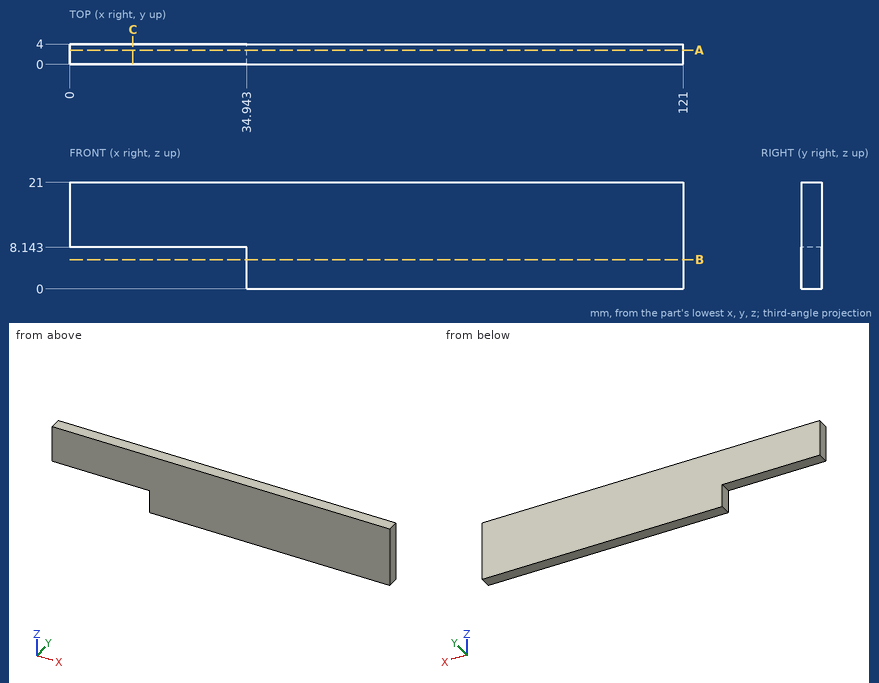
Here's the drawing with two shaded views (mm, measured from the low corner). I have some questions. Coordinates: 2 decimals unless noted, no trailing zeros. Write each loop counter-clockwise with the first axis right and the second up, starting at its lowest first coordinate (ties: lowest second). Pieces come first, ordered by that corner, then holes. Notation, with made-up numbers: M 20,41 L 57,41 A10 cw 57,59 Z; hole C 37,54 d5. An arc over 180 degrees is marked long. Write item = value, one per line. Start each with the question number.
Q1. If we section it at A-A, the plane y = 2.8: Write out the boundary of the cut face in (x, z).
Q2. If we section it at C-C, the plane x = 12.5: Write out the boundary of the cut face in (y, z).
Q3. If I drill on L1, parallel to X at y = 0.4, z = 6.5; L2, parallel to Z at x = 22, y = 0.55, over which ranges is the centre line in solid material (lowest first)? Write a range as [from, to].
Q4. If we section it at B-B, the plane z = 5.75: Write out the boundary of the cut face in (x, y).
Q5. I'm going to push a flat-ended pin straight in: pin 1 (2 mm diameter, centred on x = 28.5, y = 2, fed in from -Z). Where does the tip first touch, or does it pass through?
Check sheet entries:
q1.outline = M 0,8.14 L 34.94,8.14 L 34.94,0 L 121,0 L 121,21 L 0,21 Z
q2.outline = M 0,8.14 L 4,8.14 L 4,21 L 0,21 Z
q3.L1 = [34.94, 121]
q3.L2 = [8.14, 21]
q4.outline = M 34.94,0 L 121,0 L 121,4 L 34.94,4 Z
q5.pin_1 = 8.14
